from build123d import *

# Parameters (mm, degrees)
F1_DEPTH       = 3
F3_D           = 4.3
F3_CSINK_D     = 9
F3_CSINK_ANGLE = 90
F4_SIZE        = 1


# Not quite as in the source:
# - a feature names something its author has since deleted; it is built from what else it names


with BuildPart() as f1:
    # F0 (on Front) → F1 (new body)
    with BuildSketch(Plane.XZ):
        Polygon((0, -46.1), (0, 0), (-525, 0), (-525, -143), (0, -143), (0, -96.9), (-10, -96.9), (-10, -46.1), align=None)
    extrude(amount=F1_DEPTH)

    # F3 (through all)
    with Locations(Plane(origin=(0, 0, 0), x_dir=(1, 0, 0), z_dir=(0, 1, 0))):
        with Locations((-472.5, 5), (-332.5, 5), (-192.5, 5), (-52.5, 5), (-52.5, 138), (-192.5, 138), (-332.5, 138), (-472.5, 138)):
            CounterSinkHole(F3_D / 2, F3_CSINK_D / 2, counter_sink_angle=F3_CSINK_ANGLE)

    # F4
    f4_edges = [f1.edges().sort_by_distance(p)[0] for p in [
        (-525, -1.5, 0),
        (-525, -1.5, -143),
        (0, -1.5, -143),
        (0, -1.5, 0),
    ]]
    chamfer(f4_edges, length=F4_SIZE)


solid = f1.part
Check sheet for the modelled part. Datum: model origin and axes. Units: mm. Round coordinates to 2 decimals unless told otherwise and drop trailing zeros. Write each loop counter-clockwise with the first axis right and the second up, starting at its lowest first coordinate (ties: lowest second). Pieces come first, ordered by that corner, then holes. Notation, with made-up numbers: (6.25, 20.5) - (19.25, 20.5) arc R10 cw to (19.25, 25.5) - close; hole circle Ø8 at (-4, -20). An arc over 180 degrees is marked (long way). Return JSON: item names as keys, results as strings.
Q1. Depth check by flat-ended pin: P1, Ø7, axis at x = -472.5, z = -138, coming from the +Y side. Enter the tip coordinate at first touch or a pass-through.
Returned:
{"P1": "stops at y = -1"}
Q2. Draft check along Z on faces 1 (the flat face through (-266, -3, -70)), 2 (the conical face through (-330.703, -2.236, -3.622)), 3 (the conical face through (-470.703, -2.236, -136.622)). Enter one of: released by +Z, released by -Z, zero draft, split by the parting line, or undercut.
Returned:
{"face 1": "zero draft", "face 2": "undercut", "face 3": "undercut"}
Q3. Scan lines: L1, parallel to X at y = -2.75, z = -138; L2, parallel to Z at x = -472.5, y = -2.7; L3, parallel to X at y = -1.15, z = -5.5. Record each from-to range of solid material in increasing order. Write a range as from..to.
Returned:
{"L1": "x = -525..-474.65, -470.35..-334.65, -330.35..-194.65, -190.35..-54.65, -50.35..0", "L2": "z = -143..-140.15, -135.85..-7.15, -2.85..0", "L3": "x = -525..-475.81, -469.19..-335.81, -329.19..-195.81, -189.19..-55.81, -49.19..0"}
Q4. Cross-section at A-A (z = -71.5). Record the boundary of the cut face in (x, y).
Returned:
{"outline": "(-525, -3) - (-10, -3) - (-10, 0) - (-525, 0) - close"}
